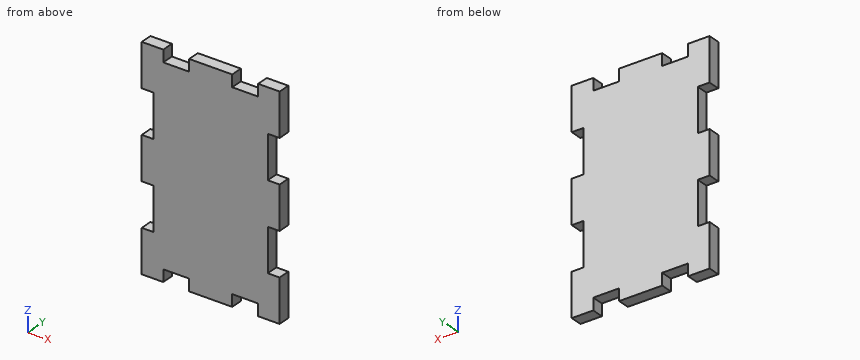
Autodesk Inventor part; units mm, degrees
ref_plane "YZ Plane" through (0, 0, 0) normal (1, 0, 0) x (0, 1, 0)
ref_plane "XZ Plane" through (0, 0, 0) normal (0, 1, 0) x (-1, 0, 0)
ref_plane "XY Plane" through (0, 0, 0) normal (0, 0, 1) x (1, 0, 0)
sketch "Block1" plane through (0, 0, 0) normal (0, 0, 1) x (1, 0, 0)
  line L0 (-10.1, 50.1) -> (-10.1, 41.1)
  line L1 (-10.1, 41.1) -> (-21.9, 41.1)
  line L2 (-21.9, 41.1) -> (-21.9, 50.1)
  line L3 (-21.9, 50.1) -> (-35.6, 50.1)
  line L4 (-35.6, 50.1) -> (-35.6, 29.9)
  line L5 (-35.6, 29.9) -> (-26.6, 29.9)
  line L6 (-26.6, 29.9) -> (-26.6, 10.1)
  line L7 (-26.6, 10.1) -> (-35.6, 10.1)
  line L8 (-35.6, 10.1) -> (-35.6, -10.1)
  line L9 (-35.6, -10.1) -> (-26.6, -10.1)
  line L10 (-26.6, -10.1) -> (-26.6, -29.9)
  line L11 (-26.6, -29.9) -> (-35.6, -29.9)
  line L12 (-35.6, -29.9) -> (-35.6, -50.1)
  line L13 (-35.6, -50.1) -> (-21.9, -50.1)
  line L14 (-21.9, -50.1) -> (-21.9, -41.1)
  line L15 (-21.9, -41.1) -> (-10.1, -41.1)
  line L16 (-10.1, -41.1) -> (-10.1, -50.1)
  line L17 (-10.1, -50.1) -> (10.1, -50.1)
  line L18 (10.1, -50.1) -> (10.1, -41.1)
  line L19 (10.1, -41.1) -> (21.9, -41.1)
  line L20 (21.9, -41.1) -> (21.9, -50.1)
  line L21 (21.9, -50.1) -> (35.6, -50.1)
  line L22 (35.6, -50.1) -> (35.6, -29.9)
  line L23 (35.6, -29.9) -> (26.6, -29.9)
  line L24 (26.6, -29.9) -> (26.6, -10.1)
  line L25 (26.6, -10.1) -> (35.6, -10.1)
  line L26 (35.6, -10.1) -> (35.6, 10.1)
  line L27 (35.6, 10.1) -> (26.6, 10.1)
  line L28 (26.6, 10.1) -> (26.6, 29.9)
  line L29 (26.6, 29.9) -> (35.6, 29.9)
  line L30 (35.6, 29.9) -> (35.6, 50.1)
  line L31 (35.6, 50.1) -> (21.9, 50.1)
  line L32 (21.9, 50.1) -> (21.9, 41.1)
  line L33 (21.9, 41.1) -> (10.1, 41.1)
  line L34 (10.1, 41.1) -> (10.1, 50.1)
  line L35 (10.1, 50.1) -> (-10.1, 50.1)
  point P0 (0, 0)
sketch "Block2" plane through (0, 0, 0) normal (0, 0, 1) x (1, 0, 0)
  line L0 (-10.2, 50.2) -> (-10.2, 41.2)
  line L1 (-10.2, 41.2) -> (-21.8, 41.2)
  line L2 (-21.8, 41.2) -> (-21.8, 50.2)
  line L3 (-21.8, 50.2) -> (-35.7, 50.2)
  line L4 (-35.7, 50.2) -> (-35.7, 29.8)
  line L5 (-35.7, 29.8) -> (-26.7, 29.8)
  line L6 (-26.7, 29.8) -> (-26.7, 10.2)
  line L7 (-26.7, 10.2) -> (-35.7, 10.2)
  line L8 (-35.7, 10.2) -> (-35.7, -10.2)
  line L9 (-35.7, -10.2) -> (-26.7, -10.2)
  line L10 (-26.7, -10.2) -> (-26.7, -29.8)
  line L11 (-26.7, -29.8) -> (-35.7, -29.8)
  line L12 (-35.7, -29.8) -> (-35.7, -50.2)
  line L13 (-35.7, -50.2) -> (-21.8, -50.2)
  line L14 (-21.8, -50.2) -> (-21.8, -41.2)
  line L15 (-21.8, -41.2) -> (-10.2, -41.2)
  line L16 (-10.2, -41.2) -> (-10.2, -50.2)
  line L17 (-10.2, -50.2) -> (10.2, -50.2)
  line L18 (10.2, -50.2) -> (10.2, -41.2)
  line L19 (10.2, -41.2) -> (21.8, -41.2)
  line L20 (21.8, -41.2) -> (21.8, -50.2)
  line L21 (21.8, -50.2) -> (35.7, -50.2)
  line L22 (35.7, -50.2) -> (35.7, -29.8)
  line L23 (35.7, -29.8) -> (26.7, -29.8)
  line L24 (26.7, -29.8) -> (26.7, -10.2)
  line L25 (26.7, -10.2) -> (35.7, -10.2)
  line L26 (35.7, -10.2) -> (35.7, 10.2)
  line L27 (35.7, 10.2) -> (26.7, 10.2)
  line L28 (26.7, 10.2) -> (26.7, 29.8)
  line L29 (26.7, 29.8) -> (35.7, 29.8)
  line L30 (35.7, 29.8) -> (35.7, 50.2)
  line L31 (35.7, 50.2) -> (21.8, 50.2)
  line L32 (21.8, 50.2) -> (21.8, 41.2)
  line L33 (21.8, 41.2) -> (10.2, 41.2)
  line L34 (10.2, 41.2) -> (10.2, 50.2)
  line L35 (10.2, 50.2) -> (-10.2, 50.2)
  point P0 (0, 0)
sketch "Block3" plane through (0, 0, 0) normal (0, 0, 1) x (1, 0, 0)
  line L0 (-10.1, 50.1) -> (-10.1, 41.1)
  line L1 (-10.1, 41.1) -> (-21.9, 41.1)
  line L2 (-21.9, 41.1) -> (-21.9, 50.1)
  line L3 (-21.9, 50.1) -> (-35.6, 50.1)
  line L4 (-35.6, 50.1) -> (-35.6, 29.9)
  line L5 (-35.6, 29.9) -> (-26.6, 29.9)
  line L6 (-26.6, 29.9) -> (-26.6, 10.1)
  line L7 (-26.6, 10.1) -> (-35.6, 10.1)
  line L8 (-35.6, 10.1) -> (-35.6, -10.1)
  line L9 (-35.6, -10.1) -> (-26.6, -10.1)
  line L10 (-26.6, -10.1) -> (-26.6, -29.9)
  line L11 (-26.6, -29.9) -> (-35.6, -29.9)
  line L12 (-35.6, -29.9) -> (-35.6, -50.1)
  line L13 (-35.6, -50.1) -> (-21.9, -50.1)
  line L14 (-21.9, -50.1) -> (-21.9, -41.1)
  line L15 (-21.9, -41.1) -> (-10.1, -41.1)
  line L16 (-10.1, -41.1) -> (-10.1, -50.1)
  line L17 (-10.1, -50.1) -> (10.1, -50.1)
  line L18 (10.1, -50.1) -> (10.1, -41.1)
  line L19 (10.1, -41.1) -> (21.9, -41.1)
  line L20 (21.9, -41.1) -> (21.9, -50.1)
  line L21 (21.9, -50.1) -> (35.6, -50.1)
  line L22 (35.6, -50.1) -> (35.6, -29.9)
  line L23 (35.6, -29.9) -> (26.6, -29.9)
  line L24 (26.6, -29.9) -> (26.6, -10.1)
  line L25 (26.6, -10.1) -> (35.6, -10.1)
  line L26 (35.6, -10.1) -> (35.6, 10.1)
  line L27 (35.6, 10.1) -> (26.6, 10.1)
  line L28 (26.6, 10.1) -> (26.6, 29.9)
  line L29 (26.6, 29.9) -> (35.6, 29.9)
  line L30 (35.6, 29.9) -> (35.6, 50.1)
  line L31 (35.6, 50.1) -> (21.9, 50.1)
  line L32 (21.9, 50.1) -> (21.9, 41.1)
  line L33 (21.9, 41.1) -> (10.1, 41.1)
  line L34 (10.1, 41.1) -> (10.1, 50.1)
  line L35 (10.1, 50.1) -> (-10.1, 50.1)
  point P0 (0, 0)
sketch "Block4" plane through (0, 0, 0) normal (0, 0, 1) x (1, 0, 0)
  line L0 (-10.08, 50.08) -> (-10.08, 44.58)
  line L1 (-10.08, 44.58) -> (-21.92, 44.58)
  line L2 (-21.92, 44.58) -> (-21.92, 50.08)
  line L3 (-21.92, 50.08) -> (-32.08, 50.08)
  line L4 (-32.08, 50.08) -> (-32.08, 29.92)
  line L5 (-32.08, 29.92) -> (-26.58, 29.92)
  line L6 (-26.58, 29.92) -> (-26.58, 10.08)
  line L7 (-26.58, 10.08) -> (-32.08, 10.08)
  line L8 (-32.08, 10.08) -> (-32.08, -10.08)
  line L9 (-32.08, -10.08) -> (-26.58, -10.08)
  line L10 (-26.58, -10.08) -> (-26.58, -29.92)
  line L11 (-26.58, -29.92) -> (-32.08, -29.92)
  line L12 (-32.08, -29.92) -> (-32.08, -50.08)
  line L13 (-32.08, -50.08) -> (-21.92, -50.08)
  line L14 (-21.92, -50.08) -> (-21.92, -44.58)
  line L15 (-21.92, -44.58) -> (-10.08, -44.58)
  line L16 (-10.08, -44.58) -> (-10.08, -50.08)
  line L17 (-10.08, -50.08) -> (10.08, -50.08)
  line L18 (10.08, -50.08) -> (10.08, -44.58)
  line L19 (10.08, -44.58) -> (21.92, -44.58)
  line L20 (21.92, -44.58) -> (21.92, -50.08)
  line L21 (21.92, -50.08) -> (32.08, -50.08)
  line L22 (32.08, -50.08) -> (32.08, -29.92)
  line L23 (32.08, -29.92) -> (26.58, -29.92)
  line L24 (26.58, -29.92) -> (26.58, -10.08)
  line L25 (26.58, -10.08) -> (32.08, -10.08)
  line L26 (32.08, -10.08) -> (32.08, 10.08)
  line L27 (32.08, 10.08) -> (26.58, 10.08)
  line L28 (26.58, 10.08) -> (26.58, 29.92)
  line L29 (26.58, 29.92) -> (32.08, 29.92)
  line L30 (32.08, 29.92) -> (32.08, 50.08)
  line L31 (32.08, 50.08) -> (21.92, 50.08)
  line L32 (21.92, 50.08) -> (21.92, 44.58)
  line L33 (21.92, 44.58) -> (10.08, 44.58)
  line L34 (10.08, 44.58) -> (10.08, 50.08)
  line L35 (10.08, 50.08) -> (-10.08, 50.08)
  point P0 (0, 0)
sketch "Sketch1" plane through (0, 0, 0) normal (0, 1, 0) x (-1, 0, 0)
  line L0 (32, -50) -> (-32, -50)
  line L1 (-32, -50) -> (-32, 50)
  line L2 (-32, 50) -> (32, 50)
  line L3 (32, 50) -> (32, -50)
  line L4 (32, -50) -> (-32, 50) construction
  line L5 (-32, -50) -> (32, 50) construction
  point P0 (0, 0)
  dimension "d0" = 64
  dimension "d1" = 100
extrude "Extrusion1" add sketch "Sketch1" along normal blind 5.5
sketch "Sketch5" plane through (0, 5.5, 0) normal (0, 1, 0) x (1, 0, 0)
  line L0 (32, 50) -> (-32, 50)
  line L1 (-32, 50) -> (-32, -50)
  line L2 (-32, 30) -> (-26.5, 30)
  line L3 (-26.5, 30) -> (-26.5, 10)
  line L4 (-26.5, 10) -> (-32, 10)
  line L5 (-32, 10) -> (-32, 30)
  line L6 (-66.1027, 0) -> (147.4162, 0)
  line L7 (0, 70.495) -> (0, -72.2701)
  line L8 (-32, -30) -> (-26.5, -30)
  line L9 (-26.5, -30) -> (-26.5, -10)
  line L10 (-26.5, -10) -> (-32, -10)
  line L11 (-32, -10) -> (-32, -30)
  line L12 (32, 30) -> (26.5, 30)
  line L13 (26.5, 30) -> (26.5, 10)
  line L14 (26.5, 10) -> (32, 10)
  line L15 (32, 10) -> (32, 30)
  line L16 (32, -30) -> (26.5, -30)
  line L17 (26.5, -30) -> (26.5, -10)
  line L18 (26.5, -10) -> (32, -10)
  line L19 (32, -10) -> (32, -30)
  point P0 (0, 0)
  dimension "d12" = 20
  dimension "d13" = 20
  dimension "d14" = 5.5
extrude "Extrusion3" cut sketch "Sketch5" against normal through all contours L10 L9 L8 L1 | L2 L3 L4 L1 | L15 L14 L13 L12 | L16 L17 L18 L19
sketch "Sketch6" plane through (0, 5.5, 0) normal (0, 1, 0) x (1, 0, 0)
  line L0 (32, 50) -> (-32, 50)
  line L1 (-66.1027, 0) -> (147.4162, 0)
  line L2 (0, 70.495) -> (0, -72.2701)
  line L3 (-22, 50) -> (-10, 50)
  line L4 (-10, 50) -> (-10, 44.5)
  line L5 (-10, 44.5) -> (-22, 44.5)
  line L6 (-22, 44.5) -> (-22, 50)
  line L7 (22, 50) -> (10, 50)
  line L8 (10, 50) -> (10, 44.5)
  line L9 (10, 44.5) -> (22, 44.5)
  line L10 (22, 44.5) -> (22, 50)
  line L11 (-22, -50) -> (-10, -50)
  line L12 (-10, -50) -> (-10, -44.5)
  line L13 (-10, -44.5) -> (-22, -44.5)
  line L14 (-22, -44.5) -> (-22, -50)
  line L15 (10, -44.5) -> (22, -44.5)
  line L16 (22, -50) -> (10, -50)
  line L17 (10, -50) -> (10, -44.5)
  line L18 (22, -44.5) -> (22, -50)
  point P0 (0, 0)
  dimension "d17" = 5.5
  dimension "d18" = 12
  dimension "d19" = 20
extrude "Extrusion4" cut sketch "Sketch6" against normal through all
equation "\"d2\" = Wt"
equation "\"d14\" = Wt"
equation "\"d15\" = Wt"
equation "\"d17\" = Wt"
equation "\"d20\" = Wt"
properties part number "holder_ceil_plate" material "Wood (Birch)"
Can you work these out from the model? Positions are in its coordinate system, mm. Give positions to 0.01 mm unless a question says otherwise; leave off trailing zeros. Loops run counter-clockwise (first coordinate to the right, second up) from the corner with the lowest first, then second, coordinate; pieces in that order, holes last. Notation, with made-up numbers: M -20,7.25 L 32,7.25 A23 cw 32,21.25 Z; hole C 81,30.5 d5. An arc over 180 degrees is marked long. Answer in a Markdown table with one row per item.
1. Suppose I cut it at B-B on x = -15. Write out the boundary of the cut face in (y, z), plus the area to 4 significant figures.
Taken from the geometry:
| item | result |
|---|---|
| outline | M 0,-44.5 L 5.5,-44.5 L 5.5,44.5 L 0,44.5 Z |
| area | 489.5 mm² |
2. Suppose I cut it at A-A on x = 28. Write out the boundary of the cut face in (y, z).
Taken from the geometry:
| item | result |
|---|---|
| outline | M 0,-50 L 5.5,-50 L 5.5,-30 L 0,-30 Z; M 0,-10 L 5.5,-10 L 5.5,10 L 0,10 Z; M 0,30 L 5.5,30 L 5.5,50 L 0,50 Z |
3. Suppose I cut it at C-C on z = 17.5. Write out the boundary of the cut face in (x, y).
Taken from the geometry:
| item | result |
|---|---|
| outline | M -26.5,0 L 26.5,0 L 26.5,5.5 L -26.5,5.5 Z |
4. If I drill on line 1 along X through (y, z) = (4.6, 45); line 2 along Z through (x, y) = (-27, 0.65); line 3 along Z through (x, y) = (19, 3), over which ranges is the centre line in solid material (lowest first)?
Taken from the geometry:
| item | result |
|---|---|
| line 1 | x = -32 to -22, -10 to 10, 22 to 32 |
| line 2 | z = -50 to -30, -10 to 10, 30 to 50 |
| line 3 | z = -44.5 to 44.5 |
5. For pin 1 Ø3 at (y, z) = (2.5, -21.5) entering from -X; pin 2 Ø1.5 at (x, y) = (-11, 2) entering from +Z; pin 3 Ø6 at (x, z) = (8, -36.5) entering from -Y, each with a flat end and sliding along its axis, tell me the tip position at first contact or that it passes through.
Taken from the geometry:
| item | result |
|---|---|
| pin 1 | stops at x = -26.5 |
| pin 2 | stops at z = 44.5 |
| pin 3 | stops at y = 0 |
